```python
from build123d import *

# Parameters (mm, degrees)
EXTRUDE_1_DEPTH     = 13
CUT_EXTRUDE_1_DEPTH = 11


with BuildPart() as part:
    # 草图1 → 凸台-拉伸1 (new body)
    with BuildSketch(Plane(origin=(0, 0, 0), x_dir=(1, 0, 0), z_dir=(0, 1, 0))):
        Polygon((0, 0), (0, 25), (-32, 25), (-32, 10), (-47, 10), (-47, 0), align=None)
    extrude(amount=EXTRUDE_1_DEPTH)

    # 草图2 → 切除-拉伸1 (cut)
    with BuildSketch(Plane.XZ):
        Polygon((-2, -2), (-45, -2), (-45, -8), (-30, -8), (-30, -23), (-2, -23), align=None)
    extrude(amount=-CUT_EXTRUDE_1_DEPTH, mode=Mode.SUBTRACT)


solid = part.part
```
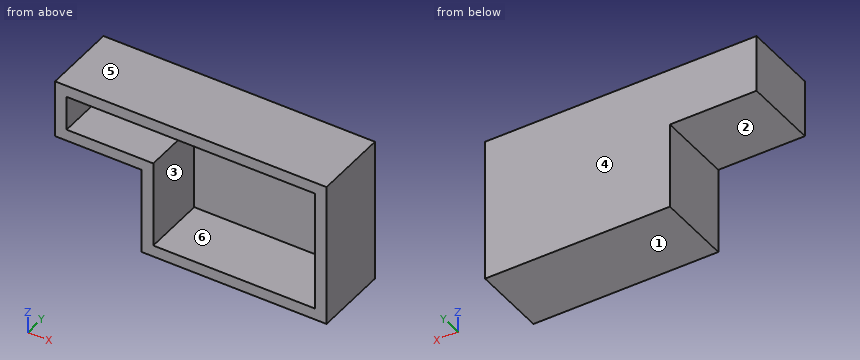
The listing builds one solid part. Answer for the finished solid, in the listing's coordinates (mm). Face numbers are marked on the shaded views. A direction names the side the tool comes from. Round coordinates to 2 decimals unless told otherwise and drop trailing zeros. Loops run counter-clockwise (first coordinate to the right, second up) from the corner with the lowest first, then second, coordinate; pieces in that order, holes last.
1) For a pull along Z with two mould halves and no side action, classify the marked faces 4, 5 and 6 as released by +Z, released by -Z, zero draft, split by the parting line, or undercut.
Outcome:
face 4: zero draft
face 5: released by +Z
face 6: undercut
2) For the marked faces 1, 2 and 3, determine the directions among +Z, -Z, +X, -X, +Y, -Y from which every point of the face is accessible in a straight line to the end or side of a thin tool.
Outcome:
face 1: -Z, +X, -X, +Y, -Y
face 2: -Z, -X, +Y, -Y
face 3: -Y
3) A cutting plane is placed at A-A on x = -37. Determine the outline of the cut face in (y, z), plus the area to 3 significant figures.
Outcome:
outline: (0, -10) - (13, -10) - (13, 0) - (0, 0) - (0, -2) - (11, -2) - (11, -8) - (0, -8) - close
area: 64.0 mm2
4) A cutting plane is placed at D-D on y = 11.75. Determine the outline of the cut face in (x, z), plus the area to 3 significant figures.
Outcome:
outline: (-47, -10) - (-32, -10) - (-32, -25) - (0, -25) - (0, 0) - (-47, 0) - close
area: 950 mm2
5) Given P1, Ø2, axis at y = 3.5, z = -19.5, coming from the -X side, flat-ended and moving along its own axis, determine where the tip first touches the part or whether it passes through.
Outcome:
P1: stops at x = -32
6) A cutting plane is placed at C-C on y = 2.5. Determine the outline of the cut face in (x, z).
Outcome:
outline: (-47, -10) - (-32, -10) - (-32, -25) - (0, -25) - (0, 0) - (-47, 0) - close; hole (-45, -8) - (-30, -8) - (-30, -23) - (-2, -23) - (-2, -2) - (-45, -2) - close
7) A cutting plane is placed at B-B on z = -15.5. Determine the outline of the cut face in (x, y), plus the area to 3 significant figures.
Outcome:
outline: (-32, 0) - (-30, 0) - (-30, 11) - (-2, 11) - (-2, 0) - (0, 0) - (0, 13) - (-32, 13) - close
area: 108 mm2
8) Consider line 1 (X direction, y = 5, z = -4.75); line 2 (Z direction, x = -8, y = 7); line 3 (X direction, y = 6, z = -21.25). Determine where each line is inside the solid, lowest interval first.
Outcome:
line 1: x = -47 to -45, -2 to 0
line 2: z = -25 to -23, -2 to 0
line 3: x = -32 to -30, -2 to 0
